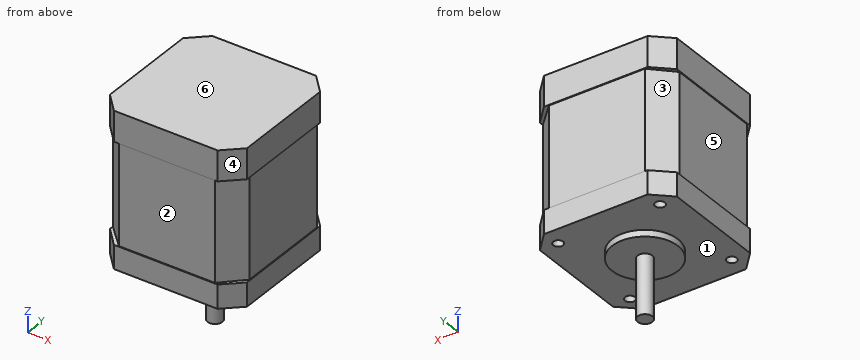
```python
from build123d import *

# Parameters (mm, degrees)
RESSALTO_EXTRUS_O1_DEPTH   = 47
CORTE_EXTRUS_O_FINA1_START = -39.8
CORTE_EXTRUS_O_FINA1_DEPTH = 30.6
ESBO_O3_R                  = 2.25
RESSALTO_EXTRUS_O2_DEPTH   = 20
ESBO_O4_R                  = 10
RESSALTO_EXTRUS_O3_DEPTH   = 2
ESBO_O5_R                  = 1.5
CORTE_EXTRUS_O1_DEPTH      = 10


# Read off the part's stored shape, not the designer's step: Corte-Extrusão-Fina1
with BuildPart() as part:
    # Esboço1 → Ressalto-extrusão1 (new body)
    with BuildSketch(Plane.XY):
        Polygon((-21, -15.592171873), (-15.984175996, -21), (15.592171873, -21), (21, -15.984175996), (21, 15.592171873), (15.984175996, 21), (-15.592171873, 21), (-21, 15.984175996), align=None)
    extrude(amount=RESSALTO_EXTRUS_O1_DEPTH)

    # Corte-Extrusão-Fina1 outline → Corte-Extrusão-Fina1 (cut)
    with BuildSketch(Plane.XY.offset(47).offset(CORTE_EXTRUS_O_FINA1_START)):
        Polygon((15.592171873, -21), (21, -15.984175996), (21, 15.592171873), (15.984175996, 21), (-15.592171873, 21), (-21, 15.984175996), (-21, -15.592171873), (-15.984175996, -21), align=None)
        Polygon((14.605339059, 20.75), (20.75, 14.605339059), (20.75, -14.605339059), (14.605339059, -20.75), (-14.605339059, -20.75), (-20.75, -14.605339059), (-20.75, 14.605339059), (-14.605339059, 20.75), align=None, mode=Mode.SUBTRACT)
    extrude(amount=CORTE_EXTRUS_O_FINA1_DEPTH, mode=Mode.SUBTRACT)

    # Esboço3 → Ressalto-extrusão2 (add)
    with BuildSketch(Plane(origin=(0, 0, 0), x_dir=(-1, 0, 0), z_dir=(0, 0, -1))):
        with Locations(Location((0, 0, 0), (0, 0, 180))):
            Circle(ESBO_O3_R)
    extrude(amount=RESSALTO_EXTRUS_O2_DEPTH)

    # Esboço4 → Ressalto-extrusão3 (add)
    with BuildSketch(Plane(origin=(0, 0, 0), x_dir=(-1, 0, 0), z_dir=(0, 0, -1))):
        with Locations(Location((0, 0, 0), (0, 0, 180))):
            Circle(ESBO_O4_R)
    extrude(amount=RESSALTO_EXTRUS_O3_DEPTH)

    # Esboço5 → Corte-extrusão1 (cut)
    with BuildSketch(Plane(origin=(0, 0, 0), x_dir=(-1, 0, 0), z_dir=(0, 0, -1))):
        with Locations((15.5, -15.5)):
            Circle(ESBO_O5_R)
        with Locations((-15.5, -15.5)):
            Circle(ESBO_O5_R)
        with Locations((-15.5, 15.5)):
            Circle(ESBO_O5_R)
        with Locations((15.5, 15.5)):
            Circle(ESBO_O5_R)
    extrude(amount=-CORTE_EXTRUS_O1_DEPTH, mode=Mode.SUBTRACT)


solid = part.part
```
CAD build for the part. Positions are in the model's coordinates, mm. Face numbers are marked on the shaded views. A direction names the side the tool comes from. Give positions to 0.01 mm unless a question says otherwise; leave off trailing zeros. Loops run counter-clockwise (first coordinate to the right, second up) from the corner with the lowest first, then second, coordinate; pieces in that order, holes last. Notation, with made-up numbers: (39.25, -17.75) - (49.25, -17.75) arc R34 ccw to (49.25, 14.25) - close; hole circle Ø4 at (51.5, -7). An arc over 180 degrees is marked (long way). Put each result on its own line as item: value.
Q1. Mould opens along Z. For the marked faces 4, 5 and 6 say: pulls with the +Z half, pulls with the -Z half, needs draft (parallel to the pull), parting line crosses it, or undercut.
Filled in:
face 4: needs draft
face 5: undercut
face 6: pulls with the +Z half
Q2. Slice it at C-C (x = 0). Give the cut face in (y, z).
Filled in:
outline: (-21, 0) - (-10, 0) - (-10, -2) - (-2.25, -2) - (-2.25, -20) - (2.25, -20) - (2.25, -2) - (10, -2) - (10, 0) - (21, 0) - (21, 7.2) - (20.75, 7.2) - (20.75, 37.8) - (21, 37.8) - (21, 47) - (-21, 47) - (-21, 37.8) - (-20.75, 37.8) - (-20.75, 7.2) - (-21, 7.2) - close
Q3. Probe line 1 along X through (y, z) = (15, 6); line 2 along Z through (x, y) = (-4, -4.5). List the from-to ranges inside material, lowest first.
Filled in:
line 1: x = -21 to -16.91, -14.09 to 14.09, 16.91 to 21
line 2: z = -2 to 47
Q4. Slice it at A-A (y = 11). Give the cut face in (x, z), plus the area to 3 significant figures.
Filled in:
outline: (-21, 0) - (21, 0) - (21, 7.2) - (20.75, 7.2) - (20.75, 37.8) - (21, 37.8) - (21, 47) - (-21, 47) - (-21, 37.8) - (-20.75, 37.8) - (-20.75, 7.2) - (-21, 7.2) - close
area: 1,960 mm²
Q5. Slice it at B-B (z = 11.5). Give the cut face in (x, y), plus the area to 3 significant figures.
Filled in:
outline: (-20.75, -14.61) - (-14.61, -20.75) - (14.61, -20.75) - (20.75, -14.61) - (20.75, 14.61) - (14.61, 20.75) - (-14.61, 20.75) - (-20.75, 14.61) - close
area: 1,650 mm²
Q6. Flat gauge pins, fed straight in: pin 1 (3 mm diameter, centred on y = -6, z = 14.5, fed in from +X); pin 2 (9 mm diameter, centred on x = 0.5, z = 29.5, fed in from -Y); pin 3 (14.5 mm diameter, centred on y = -3, z = 25.5, fed in from -X); pin 4 (21 mm diameter, centred on x = -6.5, y = 6, fed in from -Z). Where does each tip first touch, or does it go through?
Filled in:
pin 1: stops at x = 20.75
pin 2: stops at y = -20.75
pin 3: stops at x = -20.75
pin 4: stops at z = -20
Q7. Tool access for the marked faces 1, 2 and 3: list every direction of +Z, -Z, +X, -X, +Y, -Y with a clear straight run to the whole face (end or side of a thin tool).
Filled in:
face 1: -Z
face 2: +X, -X, -Y
face 3: -X, +Y
